Input: part model. Units: mm. Frame: model coordinates. A direction names the side the tool comes from. Give positions to 0.01 mm unless a question says otherwise; leave off trailing zeros. Loops run counter-clockwise (first coordinate to the right, second up) from the corner with the lowest first, then second, coordinate; pieces in that order, holes last. Notation, with made-up numbers: (57.25, 36.5) - (74.25, 36.5) arc R21 cw to (74.25, 64.5) - close; hole circle Ø6 at (24.25, 22.5). An arc over 180 degrees is marked (long way). One line per question, with ' | ' between items. Start each with the question number.
from build123d import *

# Parameters (mm, degrees)
F0_W     = 30
F0_H     = 30
F0_R     = 12.5
F1_DEPTH = 65
F2_W     = 2.5
F2_H     = 15
F2_W_2   = 30
F3_DEPTH = 45
F4_R     = 4
F5_DEPTH = 30.001
F6_DEPTH = 20


with BuildPart() as f1:
    # F0 (on Top) → F1 (new body)
    with BuildSketch(Plane.XY):
        Rectangle(F0_W, F0_H)
        Circle(F0_R, mode=Mode.SUBTRACT)
        Circle(F0_R)
    extrude(amount=F1_DEPTH)

    # F2 (on face) → F3 (cut)
    with BuildSketch(Plane.XY.offset(65)):
        with Locations((16.25, 0)):
            Rectangle(F2_W, F2_H)
        Rectangle(F2_W_2, F2_H)
        with Locations((-16.25, 0)):
            Rectangle(F2_W, F2_H)
    extrude(amount=-F3_DEPTH, mode=Mode.SUBTRACT)

    # F4 (on face) → F5 (cut, through all)
    with BuildSketch(Plane.XZ.offset(15)):
        with Locations((0, 10)):
            Circle(F4_R)
        with Locations((0, 57.3658570647)):
            Circle(F4_R)
    extrude(amount=-F5_DEPTH, mode=Mode.SUBTRACT)

    # F0 (on Top) → F6 (cut, through all)
    with BuildSketch(Plane.XY):
        Circle(F0_R)
    extrude(amount=F6_DEPTH, mode=Mode.SUBTRACT)


solid = f1.part
Q1. Draft query along Z for faces 4 (the face through (-13, 0, 20)), 5 (the face through (0, 15, 32)), 6 (the face through (2.15, 13.399, 13.373)). Return one class per face: +Z half, -Z half, draft (parallel to the pull), parting line (faces both ways), or undercut.
Q2. Section A-A, the plane z = 10. Output: boundary loops of the cut face in (x, y), plus the area to 3 significant figures.
Q3. Section B-B, the plane x = 0. Output: boundary loops of the cut face in (y, z).
Q4. Access query for faces 1 (the face through (0, -9, 20)), 2 (the face through (-14, 0, 0)), 3 (the face through (13, 0, 20)). Directions: +Z, -Z, +X, -X, +Y, -Y. A direction counts if a zero-diameter tool reaches every point of the face in a straight line with its end or side. Return the directions, or none.
Q5. First-contact query: pin 1 (2.5 mm diameter, centred on x = -12, y = -3.5, fed in from +Z); pin 2 (2.5 mm diameter, centred on x = 0.5, y = 11, fed in from -Z). Flat tips, straight axial feed; report the tip coordinate or a pass-through.
Q6. Section D-D, the plane x = 11.5. Output: boundary loops of the cut face in (y, z).
Q7. Section C-C, the plane y = 0. Output: boundary loops of the cut face in (x, z).
Q8. Line query: L1, parallel to Z at x = 0, y = -14.15; L2, parallel to X at y = 0, z = 5; L3, parallel to Z at x = 0, y = 11.5. Output: solid intervals per line, ascending. Write a range as from..to.
Solved:
1) face 4: +Z half | face 5: draft | face 6: undercut
2) outline: (-15, -15) - (-4, -15) - (-4, -11.84) arc R12.5 cw to (-4, 11.84) - (-4, 15) - (-15, 15) - close; (4, -15) - (15, -15) - (15, 15) - (4, 15) - (4, 11.84) arc R12.5 cw to (4, -11.84) - close | area: 366 mm²
3) outline: (-15, 0) - (-12.5, 0) - (-12.5, 6) - (-15, 6) - close; (-15, 14) - (-12.5, 14) - (-12.5, 20) - (-7.5, 20) - (-7.5, 53.37) - (-15, 53.37) - close; (-15, 61.37) - (-7.5, 61.37) - (-7.5, 65) - (-15, 65) - close; (7.5, 20) - (12.5, 20) - (12.5, 14) - (15, 14) - (15, 53.37) - (7.5, 53.37) - close; (7.5, 61.37) - (15, 61.37) - (15, 65) - (7.5, 65) - close; (12.5, 0) - (15, 0) - (15, 6) - (12.5, 6) - close
4) face 1: -Z | face 2: -Z, +X, -X, +Y, -Y | face 3: +Z, +X, -X
5) pin 1: stops at z = 20 | pin 2: stops at z = 20
6) outline: (-15, 0) - (-4.9, 0) - (-4.9, 20) - (-7.5, 20) - (-7.5, 65) - (-15, 65) - close; (4.9, 0) - (15, 0) - (15, 65) - (7.5, 65) - (7.5, 20) - (4.9, 20) - close
7) outline: (-15, 0) - (-12.5, 0) - (-12.5, 20) - (-15, 20) - close; (12.5, 0) - (15, 0) - (15, 20) - (12.5, 20) - close
8) L1: z = 0..6, 14..53.37, 61.37..65 | L2: x = -15..-12.5, 12.5..15 | L3: z = 20..53.37, 61.37..65
